Check sheet for the drawn part. Datum: minimum x, y, z corner. Units: mm. Give positions to 0.01 mm unless a question says otherwise; leave off trailing zeros. Loops run counter-clockwise (first coordinate to the right, second up) from the corner with the lowest first, then second, coordinate; pieces in that order, holes last.
1. Cross-section at D-D, the plane x = 25. Record the cut outline in (y, z).
2. Material ranges on L1, parallel to X at y = 0.5, z = 12; L2, parallel to X at y = 0.7, z = 29.5; L3, parallel to X at y = 0.15, z = 37, recorded low to high.
3. Cross-section at A-A, the plane y = 0.75. Record the cut outline in (x, z), plus the area to 3 significant figures.
4. Go/stop test with a flat-tipped pin: pin 1 Ø1.9 at (x, z) = (5, 35.91) entering from -Y. Record where the tip stops, or that it passes through.
5. Cross-section at B-B, the plane x = 5. Record the cut outline in (y, z).
6. Cross-section at C-C, the plane z = 12. Record the cut outline in (x, y).
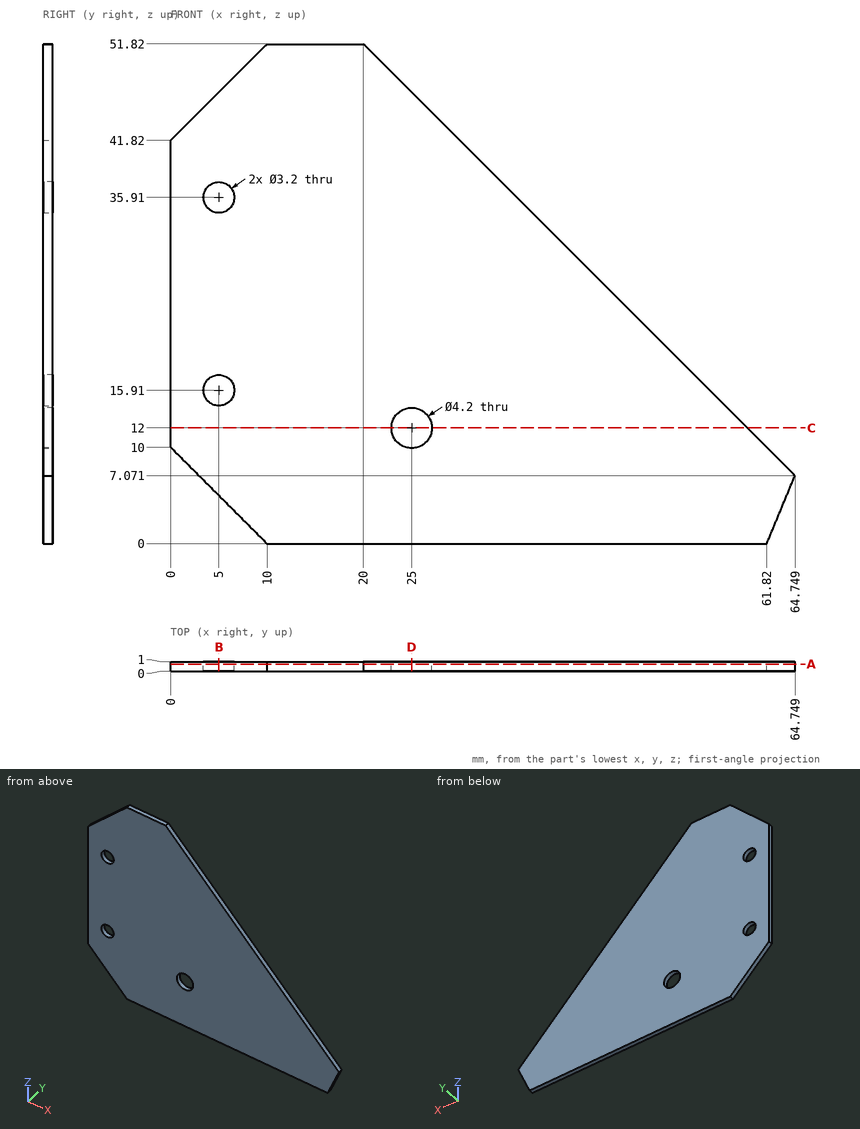
Result:
1. outline: (0, 0) - (1, 0) - (1, 9.9) - (0, 9.9) - close; (0, 14.1) - (1, 14.1) - (1, 46.82) - (0, 46.82) - close
2. L1: x = 0 to 22.9, 27.1 to 59.82
2. L2: x = 0 to 42.32
2. L3: x = 0 to 3.83, 6.17 to 34.82
3. outline: (0, 10) - (10, 0) - (61.82, 0) - (64.75, 7.07) - (20, 51.82) - (10, 51.82) - (0, 41.82) - close; hole circle Ø3.2 at (5, 15.91); hole circle Ø3.2 at (5, 35.91); hole circle Ø4.2 at (25, 12)
3. area: 2,210 mm2
4. pin 1: passes through
5. outline: (0, 5) - (1, 5) - (1, 14.31) - (0, 14.31) - close; (0, 17.51) - (1, 17.51) - (1, 34.31) - (0, 34.31) - close; (0, 37.51) - (1, 37.51) - (1, 46.82) - (0, 46.82) - close
6. outline: (0, 0) - (22.9, 0) - (22.9, 1) - (0, 1) - close; (27.1, 0) - (59.82, 0) - (59.82, 1) - (27.1, 1) - close
